Can you work these out from the drawing? Everything is in mm from the part's minimum corner. Round coordinates to 2 decimals unless told otherwise and drop trailing zeros. Loops run counter-clockwise (first coordinate to the right, second up) from the corner with the lowest first, then second, coordinate; pieces in that order, holes last. Notation, with made-up numbers: M -1.75,41.25 L 29.25,41.25 A31 ccw 29.25,73.25 Z; hole C 80,-39 d7. An arc over 180 degrees is marked long. Use a Markdown table: item, result.
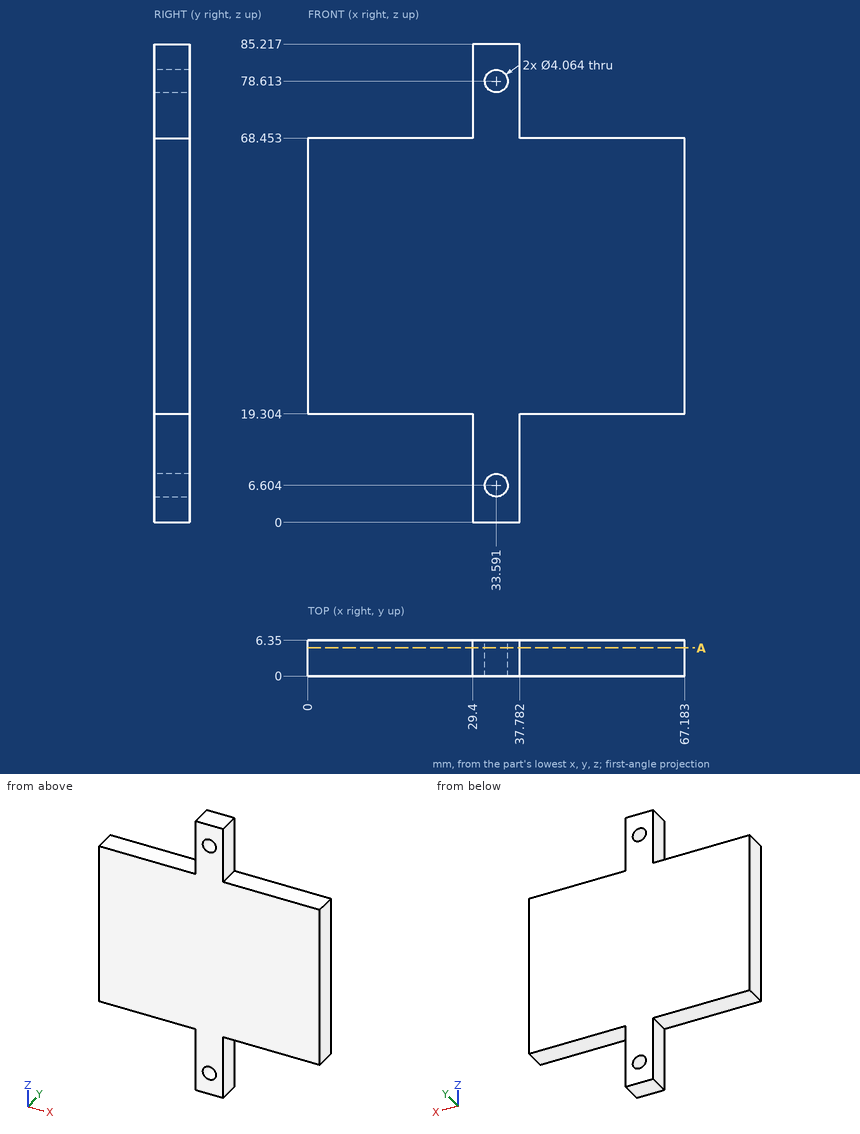
Q1. Imagine slicing it at A-A, the plane y = 5. Please give me the cut outline in (x, z) (1 decimal), then the cut area to 3 significant figures.
Return value:
| item | result |
|---|---|
| outline | M 0,19.3 L 29.4,19.3 L 29.4,0 L 37.8,0 L 37.8,19.3 L 67.2,19.3 L 67.2,68.5 L 37.8,68.5 L 37.8,85.2 L 29.4,85.2 L 29.4,68.5 L 0,68.5 Z; hole C 33.6,6.6 d4.1; hole C 33.6,78.6 d4.1 |
| area | 3,580 mm^2 |
Q2. I need wall thicknesses on line 1 (X direction, y = 1.25, z = 6.5); line 2 (Z direction, x = 50, y = 4.75) (1 decimal); line 3 (X direction, y = 6, z = 8) (1 decimal). Which ranges of each line are inside material? Lowest first, please. Write a range as from..to.
Return value:
| item | result |
|---|---|
| line 1 | x = 29.4..31.56, 35.62..37.78 |
| line 2 | z = 19.3..68.5 |
| line 3 | x = 29.4..32.1, 35.1..37.8 |
Q3. Will these pins go through, and if not, where does the flat tip stop? P1, Ø3, axis at x = 57, y = 3, coming from the -Z side; P2, Ø1.5, axis at x = 9.5, y = 4.5, coming from the +Z side; P3, Ø3, axis at y = 4.5, z = 81, coming from the +X side.
Return value:
| item | result |
|---|---|
| P1 | stops at z = 19.3 |
| P2 | stops at z = 68.45 |
| P3 | stops at x = 37.78 |
